Geometry: final body of the model. Coordinates: model frame, mm. A direction names the side the tool comes from. Give positions to 0.01 mm unless a question says otherwise; leave off trailing zeros. Loops run counter-clockwise (first coordinate to the right, second up) from the corner with the lowest first, then second, coordinate; pieces in that order, holes last.
1. Draft query along X for faces 1 (the face through (-94, -11, 30)), 2 (the face through (111.94, -5.42, -64.03)). Return one class per face: +X half, -X half, draft (parallel to the pull), parting line (faces both ways), or undercut.
2. Section A-A, the plane z = 0. Output: boundary loops of the cut face in (x, y), then the cut area to 3 significant figures.
3. Access query for faces 3 (the face through (2, 0, -30)), 4 (the face through (32.13, -10.846, 32.217)). Directions: +Z, -Z, +X, -X, +Y, -Y. A direction counts if a zero-diameter tool reaches every point of the face in a straight line with its end or side. Return the directions, or none.
4. Section B-B, the plane x = 0. Output: boundary loops of the cut face in (y, z).
5. First-contact query: P1, Ø6.5, axis at x = -68.68, z = -104.43, coming from the +Y side; P2, Ø6, axis at x = 28, z = -104, coming from the -Y side; P3, Ø3, axis at y = -18.5, z = -4.5, coming from the +X side; P4, Ø2, axis at y = -5, z = -19.5, coming from the -X side. Flat tips, straight axial feed; report the tip coordinate or a pass-through.
6. Material intervals for line 1 along X through (y, z) = (-8, 40); line 2 along Z through (x, y) = (-66, -6); line 3 along Z through (x, y) = (32.5, -19.5), sorted ascending.
from build123d import *

# Parameters (mm, degrees)
F0_R     = 144
F0_R_2   = 4
F0_R_3   = 10.1
F0_R_4   = 27.5
F0_R_5   = 6
F0_R_6   = 12.5
F3_DEPTH = 25


with BuildPart() as f2:
    # F1 (on Right) → F2 (revolve)
    with BuildSketch(Plane.YZ):
        Polygon((-22, 0), (0, 0), (0, 144), (-11, 144), (-11, 95.5), (-22, 77.5), align=None)
    revolve(axis=Axis((0, -11, 0), (0, 1, 0)))

    # F0 (on Front) → F3 (intersect)
    with BuildSketch(Plane.XZ):
        Circle(F0_R)
        with Locations((-90.914431, -85.773342)):
            Circle(F0_R_2, mode=Mode.SUBTRACT)
        with Locations((-42.749098, -117.452181)):
            Circle(F0_R_2, mode=Mode.SUBTRACT)
        with Locations((-14.510453, -124.144862)):
            Circle(F0_R_2, mode=Mode.SUBTRACT)
        with Locations((-68.683127, -104.427622)):
            Circle(F0_R_2, mode=Mode.SUBTRACT)
        with Locations((-108.244515, -62.495)):
            Circle(F0_R_2, mode=Mode.SUBTRACT)
        with Locations((-119.739109, -35.847536)):
            Circle(F0_R_2, mode=Mode.SUBTRACT)
        with Locations((-124.778537, -7.267522)):
            Circle(F0_R_2, mode=Mode.SUBTRACT)
        with Locations((-69.282032, -40)):
            Circle(F0_R_3, mode=Mode.SUBTRACT)
        with BuildLine():
            ThreePointArc((-35.355339, -28.991378), (-35.344887, -21.202779), (-27.556343, -21.234136))
            Line((-27.556343, -21.234136), (-21.738307, -27.114974))
            ThreePointArc((-21.738307, -27.114974), (-21.192382, -27.598098), (-20.715148, -28.149178))
            ThreePointArc((-20.715148, -28.149178), (-19.887922, -29.716864), (-19.602291, -31.466252))
            ThreePointArc((-19.602291, -31.466252), (-22.998539, -36.548006), (-28.99292, -35.353796))
            Line((-28.99292, -35.353796), (-35.355339, -28.991378))
        make_face(mode=Mode.SUBTRACT)
        with Locations((14.510453, -124.144862)):
            Circle(F0_R_2, mode=Mode.SUBTRACT)
        with Locations((42.749098, -117.452181)):
            Circle(F0_R_2, mode=Mode.SUBTRACT)
        with Locations((0, -80)):
            Circle(F0_R_3, mode=Mode.SUBTRACT)
        with Locations((68.683127, -104.427622)):
            Circle(F0_R_2, mode=Mode.SUBTRACT)
        with Locations((90.914431, -85.773342)):
            Circle(F0_R_2, mode=Mode.SUBTRACT)
        with Locations((69.282032, -40)):
            Circle(F0_R_3, mode=Mode.SUBTRACT)
        with BuildLine():
            ThreePointArc((28.991378, -35.355339), (21.202779, -35.344887), (21.234136, -27.556343))
            Line((21.234136, -27.556343), (27.114974, -21.738307))
            ThreePointArc((27.114974, -21.738307), (27.598098, -21.192382), (28.149178, -20.715148))
            ThreePointArc((28.149178, -20.715148), (33.916363, -20.178171), (36.966252, -25.102291))
            ThreePointArc((36.966252, -25.102291), (36.547172, -27.208057), (35.353796, -28.99292))
            Line((35.353796, -28.99292), (28.991378, -35.355339))
        make_face(mode=Mode.SUBTRACT)
        with Locations((108.244515, -62.495)):
            Circle(F0_R_2, mode=Mode.SUBTRACT)
        with Locations((119.739109, -35.847536)):
            Circle(F0_R_2, mode=Mode.SUBTRACT)
        with Locations((124.778537, -7.267522)):
            Circle(F0_R_2, mode=Mode.SUBTRACT)
        with Locations((-123.091121, 21.704286)):
            Circle(F0_R_2, mode=Mode.SUBTRACT)
        with Locations((-114.767831, 49.50601)):
            Circle(F0_R_2, mode=Mode.SUBTRACT)
        with BuildLine():
            ThreePointArc((-28.991378, 35.355339), (-22.997532, 36.547589), (-19.602291, 31.466252))
            ThreePointArc((-19.602291, 31.466252), (-20.026621, 29.347862), (-21.234136, 27.556343))
            Line((-21.234136, 27.556343), (-27.114974, 21.738307))
            ThreePointArc((-27.114974, 21.738307), (-27.598098, 21.192382), (-28.149178, 20.715148))
            ThreePointArc((-28.149178, 20.715148), (-35.614955, 21.491437), (-35.353796, 28.99292))
            Line((-35.353796, 28.99292), (-28.991378, 35.355339))
        make_face(mode=Mode.SUBTRACT)
        with Locations((-69.282032, 40)):
            Circle(F0_R_3, mode=Mode.SUBTRACT)
        with Locations((-100.257378, 74.638852)):
            Circle(F0_R_2, mode=Mode.SUBTRACT)
        with Locations((-80.342023, 95.747895)):
            Circle(F0_R_2, mode=Mode.SUBTRACT)
        with Locations((-56.09541, 111.695144)):
            Circle(F0_R_2, mode=Mode.SUBTRACT)
        with Locations((-28.824678, 121.620878)):
            Circle(F0_R_2, mode=Mode.SUBTRACT)
        Circle(F0_R_4, mode=Mode.SUBTRACT)
        with BuildLine():
            ThreePointArc((35.355339, 28.991378), (36.547589, 27.20705), (36.966252, 25.102291))
            ThreePointArc((36.966252, 25.102291), (33.557364, 20.015322), (27.556343, 21.234136))
            Line((27.556343, 21.234136), (21.738307, 27.114974))
            ThreePointArc((21.738307, 27.114974), (21.192382, 27.598098), (20.715148, 28.149178))
            ThreePointArc((20.715148, 28.149178), (21.491437, 35.614955), (28.99292, 35.353796))
            Line((28.99292, 35.353796), (35.355339, 28.991378))
        make_face(mode=Mode.SUBTRACT)
        with Locations((0, 40)):
            Circle(F0_R_5, mode=Mode.SUBTRACT)
        with Locations((69.282032, 40)):
            Circle(F0_R_3, mode=Mode.SUBTRACT)
        with Locations((123.091121, 21.704286)):
            Circle(F0_R_2, mode=Mode.SUBTRACT)
        with Locations((114.767831, 49.50601)):
            Circle(F0_R_2, mode=Mode.SUBTRACT)
        with Locations((0, 80)):
            Circle(F0_R_3, mode=Mode.SUBTRACT)
        with Locations((0, 124.99)):
            Circle(F0_R_6, mode=Mode.SUBTRACT)
        with Locations((56.09541, 111.695144)):
            Circle(F0_R_2, mode=Mode.SUBTRACT)
        with Locations((100.257378, 74.638852)):
            Circle(F0_R_2, mode=Mode.SUBTRACT)
        with Locations((80.342023, 95.747895)):
            Circle(F0_R_2, mode=Mode.SUBTRACT)
    extrude(amount=F3_DEPTH, mode=Mode.INTERSECT)


solid = f2.part
Answers below:
1. face 1: draft
1. face 2: undercut
2. outline: (-144, -11) - (-95.5, -11) - (-77.5, -22) - (-27.5, -22) - (-27.5, 0) - (-144, 0) - close; (27.5, -22) - (77.5, -22) - (95.5, -11) - (144, -11) - (144, 0) - (27.5, 0) - close
2. area: 3,860 mm2
3. face 3: +Z, -Z, +X, -X, +Y
3. face 4: +Y, -Y
4. outline: (-22, -69.9) - (0, -69.9) - (0, -27.5) - (-22, -27.5) - close; (-22, 27.5) - (0, 27.5) - (0, 34) - (-22, 34) - close; (-22, 46) - (0, 46) - (0, 69.9) - (-22, 69.9) - close; (-14.3, -90.1) - (-11, -95.5) - (-11, -144) - (0, -144) - (0, -90.1) - close; (-14.3, 90.1) - (0, 90.1) - (0, 112.49) - (-11, 112.49) - (-11, 95.5) - close; (-11, 137.49) - (0, 137.49) - (0, 144) - (-11, 144) - close
5. P1: passes through
5. P2: stops at y = -11
5. P3: stops at x = 85.56
5. P4: stops at x = -142.81
6. line 1: x = -138.33 to -79.38, -59.18 to -6, 6 to 59.18, 79.38 to 138.33
6. line 2: z = -127.98 to -107.39, -101.46 to -49.55, -30.45 to 30.45, 49.55 to 127.98
6. line 3: z = -74.84 to -31.85, -19.7 to 19.7, 31.85 to 74.84
